Here's how the part is built. I have some questions about the finished solid (model axes, mm). Face numbers are marked on the shaded views. A direction names the side the tool comes from. Coordinates: 2 decimals unless noted, no trailing zeros. Order: outer loops, then holes, each group sorted by start corner. A loop starts at its lowest first (then second) coordinate and runs counter-clockwise, first axis right, second up. Notation, with made-up numbers: (73.25, 40) - (84.25, 40) arc R24 ccw to (84.25, 50) - close; hole circle Ø3 at (86, -17). An arc over 180 degrees is marked (long way). Answer in a Markdown table with one row per item. Add a question column.
Item 1: I want a section at C-C (x = 98). Please give me the cut outline in (y, z), plus the area to 3 significant figures.
Item 2: I want a section at B-B (y = 43.5). Please give me the cut outline in (x, z), plus the area to 3 significant figures.
Item 3: I want a section at A-A (y = -25). Please give me the cut outline in (x, z).
Item 4: Will these pins go through, and if not, where does the flat tip stop? pin 1 Ø8 at (x, z) = (75, 129.9) entering from -Y; pin 2 Ø17 at (x, y) = (-167, -16) entering from +Z; pin 3 Ø22 at (x, z) = (117.5, -0.5) entering from +Y; pin 4 Ø12.5 at (y, z) = (9.5, 8) entering from -X.
Item 5: Thinking about a two-plate mould opening in X: for the marked faces 1 and 2, which applies, +X half, -X half, draft (parallel to the pull), parting line (faces both ways), or undercut?
Item 6: I want a section at D-D (y = 11). Count the separate pieces of the cut face and the enclosed holes in it, plus the area to 3 significant figures.
Item 7: On a 3-axis mill with a long thin cutter (end or side, diameter ignored), from which of +Z, -Z, +X, -X, +Y, -Y can I reach the whole of each face in a straight line? I mean the marked faces 3, 4 and 5. Say none if no direction works.
Item 8: If I drill on line 1 along Z through (x, y) = (-118.5, 11); line 2 along X through (y, z) = (7.5, 18); line 3 along Y through (x, z) = (-148.5, -124.5), over which ranges is the centre line in solid material (lowest first)? Write a range as from..to.
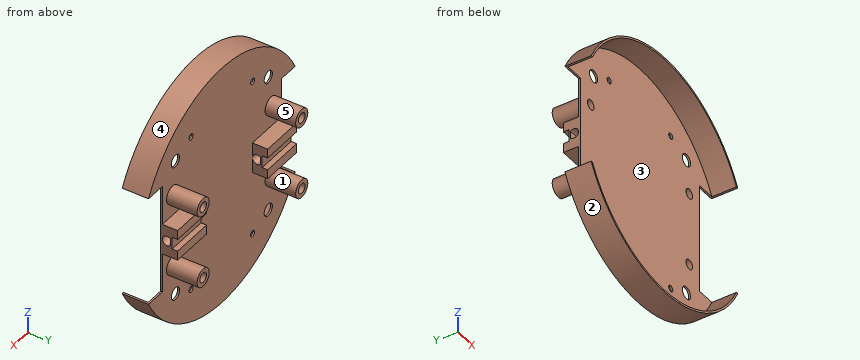
```python
from build123d import *

# Parameters (mm, degrees)
SKETCH_1_R          = 200
EXTRUDE_1_DEPTH     = 3
EXTRUDE_START       = 40
SKETCH_2_R          = 200
SKETCH_2_R_2        = 197
EXTRUDE_2_DEPTH     = 40
SKETCH_3_R          = 10
SKETCH_3_R_2        = 5
CUT_EXTRUDE_2_DEPTH = 287.092642338
SKETCH_4_W          = 70.538651056
SKETCH_4_H          = 15.178755013
EXTRUDE_4_DEPTH     = 25
SKETCH_7_W          = 70.538651056
SKETCH_7_H          = 20
EXTRUDE_5_DEPTH     = 16
CUT_EXTRUDE_5_DEPTH = 383.518831155
SKETCH_10_R         = 14.753670985
SKETCH_10_R_2       = 8
EXTRUDE_8_DEPTH     = 50
CUT_EXTRUDE_START   = -50
SKETCH_12_R         = 8
CUT_EXTRUDE_8_DEPTH = 50


with BuildPart() as part:
    # 草图1 → 凸台-拉伸1 (new body)
    with BuildSketch(Plane(origin=(0, 0, 0), x_dir=(1, 0, 0), z_dir=(0, 1, 0))):
        with Locations(Location((0, 0, 0), (0, 0, 270))):
            Circle(SKETCH_1_R)
    extrude(amount=EXTRUDE_1_DEPTH)

    # 草图2 → 凸台-拉伸2 (add)
    with BuildSketch(Plane.XZ.offset(EXTRUDE_START)):
        with Locations(Location((0, 0, 0), (0, 0, 270))):
            Circle(SKETCH_2_R)
        with Locations(Location((0, 0, 0), (0, 0, 270))):
            Circle(SKETCH_2_R_2, mode=Mode.SUBTRACT)
    extrude(amount=-EXTRUDE_2_DEPTH)

    # 草图3 → 切除-拉伸2 (cut, through all)
    with BuildSketch(Plane(origin=(0, 3, 0), x_dir=(1, 0, 0), z_dir=(0, 1, 0))):
        with BuildLine():
            ThreePointArc((200, 0), (194.577930659, 46.253960917), (178.605710995, 90))
            Line((178.605710995, 90), (145, 90))
            Line((145, 90), (145, -90))
            Line((145, -90), (178.605710995, -90))
            ThreePointArc((178.605710995, -90), (194.577930659, -46.253960917), (200, 0))
        make_face()
        with BuildLine():
            Line((-145, 90), (-178.605710995, 90))
            ThreePointArc((-178.605710995, 90), (-200, 0), (-178.605710995, -90))
            Line((-178.605710995, -90), (-145, -90))
            Line((-145, -90), (-145, 90))
        make_face()
        with Locations(Location((-113.13708499, 113.13708499, 0), (0, 0, 270))):
            Circle(SKETCH_3_R)
        with Locations(Location((-113.13708499, -113.13708499, 0), (0, 0, 270))):
            Circle(SKETCH_3_R)
        with Locations(Location((-75, 129.903810568, 0), (0, 0, 270))):
            Circle(SKETCH_3_R_2)
        with Locations(Location((113.13708499, 113.13708499, 0), (0, 0, 270))):
            Circle(SKETCH_3_R)
        with Locations(Location((75, 129.903810568, 0), (0, 0, 270))):
            Circle(SKETCH_3_R_2)
        with Locations(Location((-75, -129.903810568, 0), (0, 0, 270))):
            Circle(SKETCH_3_R_2)
        with Locations(Location((113.13708499, -113.13708499, 0), (0, 0, 270))):
            Circle(SKETCH_3_R)
        with Locations(Location((75, -129.903810568, 0), (0, 0, 270))):
            Circle(SKETCH_3_R_2)
    extrude(amount=-CUT_EXTRUDE_2_DEPTH, mode=Mode.SUBTRACT)

    # 草图4 → 凸台-拉伸4 (add)
    with BuildSketch(Plane(origin=(0, 3, 0), x_dir=(1, 0, 0), z_dir=(0, 1, 0))):
        with Locations((-109.730674472, 17.589377506)):
            Rectangle(SKETCH_4_W, SKETCH_4_H)
        with Locations((-109.730674472, -17.589377506)):
            Rectangle(SKETCH_4_W, SKETCH_4_H)
        with Locations((109.730674472, 17.589377506)):
            Rectangle(SKETCH_4_W, SKETCH_4_H)
        with Locations((109.730674472, -17.589377506)):
            Rectangle(SKETCH_4_W, SKETCH_4_H)
    extrude(amount=EXTRUDE_4_DEPTH)

    # 草图7 → 凸台-拉伸5 (add)
    with BuildSketch(Plane(origin=(0, 3, 0), x_dir=(1, 0, 0), z_dir=(0, 1, 0))):
        with Locations((-109.730674472, 0)):
            Rectangle(SKETCH_7_W, SKETCH_7_H)
        with Locations((109.730674472, 0)):
            Rectangle(SKETCH_7_W, SKETCH_7_H)
    extrude(amount=EXTRUDE_5_DEPTH)

    # 草图8 → 切除-拉伸5 (cut, through all)
    with BuildSketch(Plane.ZY.offset(145)):
        with BuildLine():
            ThreePointArc((-6.079473661, 16.2), (0, 3), (6.079473661, 16.2))
            Line((6.079473661, 16.2), (-6.079473661, 16.2))
        make_face()
    extrude(amount=-CUT_EXTRUDE_5_DEPTH, mode=Mode.SUBTRACT)

    # 草图10 → 凸台-拉伸8 (add)
    # profile 1 of 4: a face of its own
    with BuildSketch(Plane(origin=(0, 3, 0), x_dir=(1, 0, 0), z_dir=(0, 1, 0))):
        with Locations(Location((-120.048184131, 60.246329015, 0), (0, 0, 270))):
            Circle(SKETCH_10_R)
        with Locations(Location((-120.048184131, 60.246329015, 0), (0, 0, 270))):
            Circle(SKETCH_10_R_2, mode=Mode.SUBTRACT)
    # profile 2 of 4: a face of its own
    with BuildSketch(Plane(origin=(0, 3, 0), x_dir=(1, 0, 0), z_dir=(0, 1, 0))):
        with Locations(Location((-120.048184131, -60.246329015, 0), (0, 0, 270))):
            Circle(SKETCH_10_R)
        with Locations(Location((-120.048184131, -60.246329015, 0), (0, 0, 270))):
            Circle(SKETCH_10_R_2, mode=Mode.SUBTRACT)
    # profile 3 of 4: a face of its own
    with BuildSketch(Plane(origin=(0, 3, 0), x_dir=(1, 0, 0), z_dir=(0, 1, 0))):
        with Locations(Location((120.048184131, -60.246329015, 0), (0, 0, 270))):
            Circle(SKETCH_10_R)
        with Locations(Location((120.048184131, -60.246329015, 0), (0, 0, 270))):
            Circle(SKETCH_10_R_2, mode=Mode.SUBTRACT)
    # profile 4 of 4: a face of its own
    with BuildSketch(Plane(origin=(0, 3, 0), x_dir=(1, 0, 0), z_dir=(0, 1, 0))):
        with Locations(Location((120.048184131, 60.246329015, 0), (0, 0, 270))):
            Circle(SKETCH_10_R)
        with Locations(Location((120.048184131, 60.246329015, 0), (0, 0, 270))):
            Circle(SKETCH_10_R_2, mode=Mode.SUBTRACT)
    extrude(amount=EXTRUDE_8_DEPTH)

    # 草图12 → 切除-拉伸8 (cut)
    with BuildSketch(Plane(origin=(0, 3, 0), x_dir=(1, 0, 0), z_dir=(0, 1, 0)).offset(CUT_EXTRUDE_START)):
        with Locations(Location((-120.048184131, 60.246329015, 0), (0, 0, 270))):
            Circle(SKETCH_12_R)
        with Locations(Location((-120.048184131, -60.246329015, 0), (0, 0, 270))):
            Circle(SKETCH_12_R)
        with Locations(Location((120.048184131, -60.246329015, 0), (0, 0, 270))):
            Circle(SKETCH_12_R)
        with Locations(Location((120.048184131, 60.246329015, 0), (0, 0, 270))):
            Circle(SKETCH_12_R)
    extrude(amount=CUT_EXTRUDE_8_DEPTH, mode=Mode.SUBTRACT)


solid = part.part
```
Values follow:
| question | item | result |
|---|---|---|
| 1 | outline | (-40, -174.34) - (3, -174.34) - (3, -25.18) - (28, -25.18) - (28, -10) - (19, -10) - (19, 10) - (28, 10) - (28, 25.18) - (3, 25.18) - (3, 174.34) - (-40, 174.34) - (-40, 170.89) - (0, 170.89) - (0, -170.89) - (-40, -170.89) - close; hole (16.2, -6.08) - (16.2, 6.08) arc R8 ccw (long way) to start |
| 1 | area | 2,220 mm^2 |
| 2 | outline | circle Ø29.51 at (-120.05, -60.25); circle Ø29.51 at (-120.05, 60.25); circle Ø29.51 at (120.05, -60.25); circle Ø29.51 at (120.05, 60.25); hole circle Ø16 at (-120.05, -60.25); hole circle Ø16 at (-120.05, 60.25); hole circle Ø16 at (120.05, -60.25); hole circle Ø16 at (120.05, 60.25) |
| 2 | area | 1,930 mm^2 |
| 3 | outline | (-178.61, -90) arc R200 ccw to (178.61, -90) - (175.24, -90) arc R197 cw to (-175.24, -90) - close; (-178.61, 90) - (-175.24, 90) arc R197 cw to (175.24, 90) - (178.61, 90) arc R200 ccw to start |
| 4 | pin 1 | passes through |
| 4 | pin 2 | stops at z = 121.97 |
| 4 | pin 3 | stops at y = 28 |
| 4 | pin 4 | stops at x = -145 |
| 5 | face 1 | undercut |
| 5 | face 2 | parting line |
| 6 | separate pieces | 8 |
| 6 | enclosed holes | 4 |
| 6 | area | 6,780 mm^2 |
| 7 | face 3 | -Y |
| 7 | face 4 | +Z, +Y, -Y |
| 7 | face 5 | +Y |
| 8 | line 1 | z = -74.92..-68.1, -52.4..-45.57, -25.18..-8, 8..25.18, 45.57..52.4, 68.1..74.92 |
| 8 | line 2 | x = -145..-74.46, 74.46..145 |
| 8 | line 3 | y = 0..3 |
